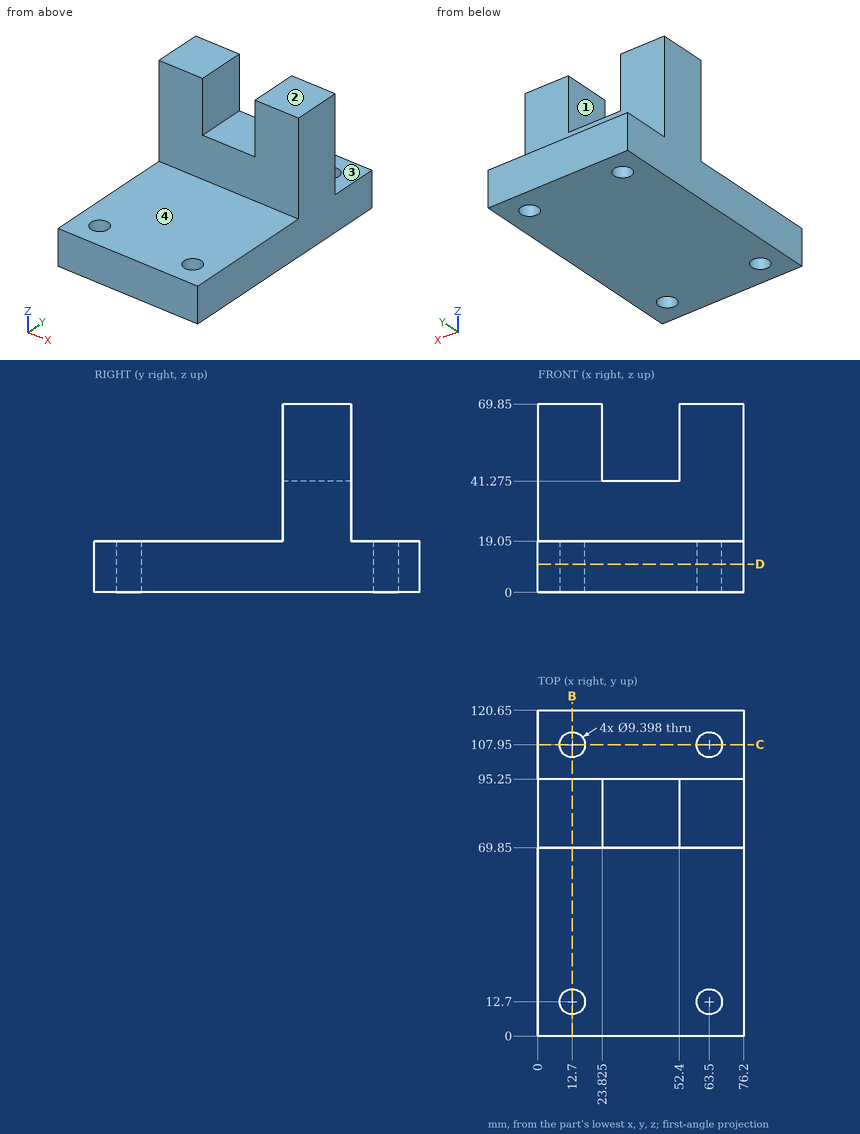
Can you work these out from the drawing? Everything is in mm from the part's minimum corner. A direction names the side the tool comes from. Coordinates: 2 decimals unless noted, no trailing zeros. Loops run counter-clockwise (first coordinate to the right, second up) from the corner with the lowest first, then second, coordinate; pieces in that order, holes last. Notation, with made-up numbers: (33.25, 75.25) - (91.25, 75.25) arc R24 cw to (91.25, 108.25) - close; hole circle Ø10 at (-9.75, 42.25). An arc over 180 degrees is marked (long way). Put each result on its own line as item: value. Start each with the question number.
Item 1: Which directions (+Z, -Z, +X, -X, +Y, -Y) give clear straight access to the entire face, cutting with the end or side of a thin tool? Please do the marked faces 1, 2, 3 and 4.
Item 2: Suppose I cut it at D-D (z = 10.5). Please give me the cut outline in (x, y).
Item 3: If I drill on line 1 along Y through (x, z) = (12.7, 12.25); line 2 along X through (y, z) = (107.95, 4.5); line 3 along X through (y, z) = (71.5, 65) (1 decimal), over which ranges is the centre line in solid material (lowest first)?
Item 4: Suppose I cut it at C-C (y = 107.95). Please give me the cut outline in (x, z).
Item 5: Suppose I cut it at B-B (x = 12.7). Please give me the cut outline in (y, z).
Item 6: For pin 1 (12 mm diameter, centred on x = 59.5, z = 54.5, fed in from +Y); pin 2 (8.5 mm diameter, centred on x = 63.5, y = 107.95, fed in from -Z); pin 3 (11 mm diameter, centred on x = 63.5, y = 12.7, fed in from +Z); pin 4 (7.5 mm diameter, centred on x = 38, y = 79.5, fed in from +Z) (3 decimals), each with a flat end and sliding along its axis, tell me the tip position at first contact or that it passes through.
Here are the results:
1. face 1: +Z, +Y, -Y
1. face 2: +Z, +X, -X, +Y, -Y
1. face 3: +Z, +X, -X, +Y
1. face 4: +Z, +X, -X, -Y
2. outline: (0, 0) - (76.2, 0) - (76.2, 120.65) - (0, 120.65) - close; hole circle Ø9.4 at (12.7, 12.7); hole circle Ø9.4 at (12.7, 107.95); hole circle Ø9.4 at (63.5, 12.7); hole circle Ø9.4 at (63.5, 107.95)
3. line 1: 0 to 8, 17.4 to 103.25, 112.65 to 120.65
3. line 2: 0 to 8, 17.4 to 58.8, 68.2 to 76.2
3. line 3: 0 to 23.8, 52.4 to 76.2
4. outline: (0, 0) - (8, 0) - (8, 19.05) - (0, 19.05) - close; (17.4, 0) - (58.8, 0) - (58.8, 19.05) - (17.4, 19.05) - close; (68.2, 0) - (76.2, 0) - (76.2, 19.05) - (68.2, 19.05) - close
5. outline: (0, 0) - (8, 0) - (8, 19.05) - (0, 19.05) - close; (17.4, 0) - (103.25, 0) - (103.25, 19.05) - (95.25, 19.05) - (95.25, 69.85) - (69.85, 69.85) - (69.85, 19.05) - (17.4, 19.05) - close; (112.65, 0) - (120.65, 0) - (120.65, 19.05) - (112.65, 19.05) - close
6. pin 1: y = 95.25
6. pin 2: through
6. pin 3: z = 19.05
6. pin 4: z = 41.275
